The listing builds one solid part. Answer for the finished solid, in the listing's coordinates (mm). Round coordinates to 2 decimals unless told otherwise and drop trailing zeros. Loops run counter-clockwise (first coordinate to the right, second up) from the corner with the lowest first, then second, coordinate; pieces in that order, holes last. Notation, with made-up numbers: (26, 45.5) -> (64, 45.5) arc R13 ccw to (64, 63.5) -> close; hole circle Ø4 at (44.25, -36.75). An arc over 180 degrees is marked (long way). Use a Markdown table: item, result. Add a question column.
Q1. Consider line 1 (Z direction, x = 4.5, y = 11); line 2 (X direction, y = -7, z = 7.25); line 3 (Y direction, x = -37, z = 24). Determine where each line is inside the solid, lowest interval first.
Q2. Section A-A on y = 9 is taken. Give the vertices of the cut face in (x, z), then the cut area to 3 significant figures.
Q3. Given pin 1 Ø3 at (y, z) = (-0.5, 21.5) entering from +X; pin 2 Ø3 at (x, y) = (32, -9) entering from +Z, each flat-ended and moving along its own axis, determine where each tip first touches the part or whether it passes through.
from build123d import *

# Parameters (mm, degrees)
SKETCH1_W           = 100.5
SKETCH1_H           = 31.15
BOSS_EXTRUDE1_DEPTH = 27
FILLET1_R           = 20
FILLET2_R           = 5


with BuildPart() as part:
    # Sketch1 → Boss-Extrude1 (new body)
    with BuildSketch(Plane.XY):
        Rectangle(SKETCH1_W, SKETCH1_H)
    extrude(amount=BOSS_EXTRUDE1_DEPTH)

    # Fillet1
    fillet1_edges = [part.edges().sort_by_distance(p)[0] for p in [
        (-50.25, 0, 27),
        (50.25, 0, 27),
    ]]
    fillet(fillet1_edges, radius=FILLET1_R)

    # Fillet2
    fillet2_edges = [part.edges().sort_by_distance(p)[0] for p in [
        (0, 15.575, 27),
        (0, -15.575, 27),
        (-50.25, 15.575, 3.5),
        (50.25, 15.575, 3.5),
        (-44.392135624, 15.575, 21.142135624),
        (44.392135624, 15.575, 21.142135624),
        (50.25, -15.575, 3.5),
        (-50.25, -15.575, 3.5),
        (-44.392135624, -15.575, 21.142135624),
        (44.392135624, -15.575, 21.142135624),
    ]]
    fillet(fillet2_edges, radius=FILLET2_R)


solid = part.part
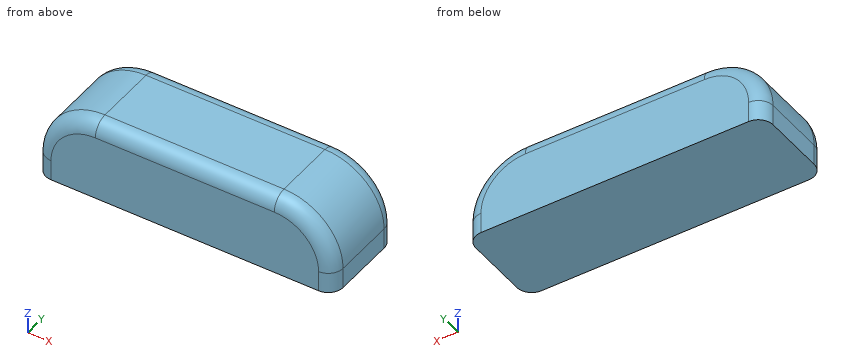
Checked values:
| question | item | result |
|---|---|---|
| 1 | line 1 | z = 0 to 26.98 |
| 1 | line 2 | x = -50.25 to 50.25 |
| 1 | line 3 | y = -14.34 to 14.34 |
| 2 | outline | (-50.25, 0) -> (50.25, 0) -> (50.25, 7) arc R20 ccw to (30.25, 27) -> (-30.25, 27) arc R20 ccw to (-50.25, 7) -> close |
| 2 | area | 2,540 mm2 |
| 3 | pin 1 | stops at x = 45.45 |
| 3 | pin 2 | stops at z = 27 |
